Input: part model. Units: mm. Frame: model coordinates. Face numbers are marked on the shaded views. A direction names the side the tool comes from. Give positions to 0.01 mm unless a question says otherwise; leave off trailing zeros. Order: outer loops, then holes, each group sorted by start corner. A loop starts at its lowest first (then second) coordinate and runs counter-clockwise, first axis right, second up. Notation, with made-up numbers: (43.5, 60.25) - (93.5, 60.25) arc R34 ccw to (93.5, 99.25) - close; hole circle Ø7 at (43, 56). An arc over 180 degrees is marked (long way). Answer in a Markdown table with one row per item. Add a question column.
1. Mould query, pull axis Z, two halves, no side actions, for the marked faces 4, 5, 6 and 7. Classes: released by +Z, released by -Z, zero draft, split by the parting line, or undercut.
2. Contact query for flat-ended pins moving along their axis: pin 1 (5 mm diameter, centred on y = 136, z = -37.5, fed in from -X); pin 2 (10 mm diameter, centred on x = -6.5, y = 178, fed in from -Z); pin 3 (4 mm diameter, centred on y = 146, z = -18, fed in from -X). Output: stop coordinate, or through.
3. Section query A-A on x = 9. Return loops of the section in (y, z).
4. Ray query, line 1 (X direction, y = 68, z = 0); line 2 (Z direction, x = 11.75, y = 40.5). Return the intervals inside material, ascending. Write a range as [from, to].
5. Access query for the marked faces 1, 2 and 3. Directions: +Z, -Z, +X, -X, +Y, -Y. A direction counts if a zero-diameter tool reaches every point of the face in a straight line with its end or side. Return the directions, or none.
6. Section query C-C on x = 0. Return loops of the section in (y, z), and give its area (3 significant figures).
7. Section query B-B on y = 25.5. Return loops of the section in (x, z).
8. Section query D-D on y = 140. Return loops of the section in (x, z), and give its area (3 significant figures).
```python
from build123d import *

# Parameters (mm, degrees)
SKETCH3_W                = 25
SKETCH3_H                = 25
SKETCH3_W_2              = 22
SKETCH3_H_2              = 22
BOSS_EXTRUDE1_DEPTH      = 200
SKETCH4_R                = 5
CUT_EXTRUDE1_DEPTH       = 25
BOSS_EXTRUDE2_DEPTH      = 55
BOSS_EXTRUDE2_DEPTH_BACK = 75
SKETCH5_R                = 5


with BuildPart() as part:
    # Sketch3 → Boss-Extrude1 (new body)
    with BuildSketch(Plane(origin=(0, 0, 0), x_dir=(1, 0, 0), z_dir=(0, 1, 0))):
        Rectangle(SKETCH3_W, SKETCH3_H)
        Rectangle(SKETCH3_W_2, SKETCH3_H_2, mode=Mode.SUBTRACT)
    extrude(amount=BOSS_EXTRUDE1_DEPTH)

    # Sketch4 → Cut-Extrude1 (cut)
    with BuildSketch(Plane.XY.offset(12.5)):
        with Locations((0, 140)):
            Circle(SKETCH4_R)
    extrude(amount=-CUT_EXTRUDE1_DEPTH, mode=Mode.SUBTRACT)

    # Sketch5 → Boss-Extrude2 (add, two sides: drawn at the far end of the back side and taken through both)
    with BuildSketch(Plane.XY.offset(-BOSS_EXTRUDE2_DEPTH_BACK)):
        with Locations((0, 140)):
            Circle(SKETCH5_R)
    extrude(amount=BOSS_EXTRUDE2_DEPTH + BOSS_EXTRUDE2_DEPTH_BACK)


solid = part.part
```
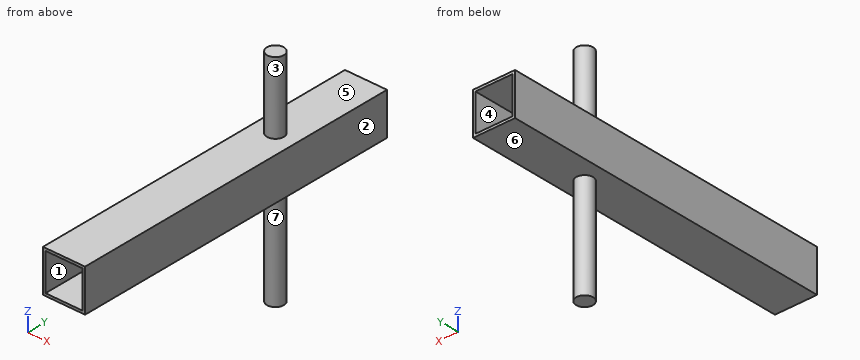
Answer:
| question | item | result |
|---|---|---|
| 1 | face 4 | undercut |
| 1 | face 5 | released by +Z |
| 1 | face 6 | released by -Z |
| 1 | face 7 | zero draft |
| 2 | pin 1 | stops at x = -4.77 |
| 2 | pin 2 | stops at z = -12.5 |
| 2 | pin 3 | stops at x = -3 |
| 3 | outline | (0, -12.5) - (200, -12.5) - (200, -11) - (0, -11) - close; (0, 11) - (200, 11) - (200, 12.5) - (0, 12.5) - close |
| 4 | line 1 | x = [-12.5, -11], [11, 12.5] |
| 4 | line 2 | z = [-12.5, 12.5] |
| 5 | face 1 | +Y, -Y |
| 5 | face 2 | +Z, -Z, +X, +Y, -Y |
| 5 | face 3 | +Z |
| 6 | outline | (0, -12.5) - (135, -12.5) - (135, -75) - (145, -75) - (145, -12.5) - (200, -12.5) - (200, -11) - (145, -11) - (145, 11) - (200, 11) - (200, 12.5) - (145, 12.5) - (145, 55) - (135, 55) - (135, 12.5) - (0, 12.5) - (0, 11) - (135, 11) - (135, -11) - (0, -11) - close |
| 6 | area | 1,870 mm² |
| 7 | outline | (-12.5, -12.5) - (12.5, -12.5) - (12.5, 12.5) - (-12.5, 12.5) - close; hole (-11, -11) - (11, -11) - (11, 11) - (-11, 11) - close |
| 8 | outline | (-12.5, -12.5) - (-5, -12.5) - (-5, -75) - (5, -75) - (5, -12.5) - (12.5, -12.5) - (12.5, 12.5) - (5, 12.5) - (5, 55) - (-5, 55) - (-5, 12.5) - (-12.5, 12.5) - close; hole (-11, -11) - (-5, -11) - (-5, 11) - (-11, 11) - close; hole (5, -11) - (11, -11) - (11, 11) - (5, 11) - close |
| 8 | area | 1,410 mm² |
